Read the model definition and answer for the solid it produces. Units are mm, in the model's axes. A direction names the side the tool comes from. Coordinates: 2 decimals unless noted, no trailing zeros. Order: outer loops, then holes, each group sorted by start corner. A loop starts at its lowest first (then second) coordinate and runs counter-clockwise, first axis right, second up. Notation, with made-up numbers: (74.5, 67) -> (82.5, 67) arc R5 cw to (82.5, 72) -> close; hole circle Ø10 at (-5, 60.25). An arc over 180 degrees is marked (long way). Return JSON: item names as keys, results as strings. Group by question number.
```python
from build123d import *

# Parameters (mm, degrees)
SKETCH1_R                                       = 28.5
BOSS_EXTRUDE1_DEPTH                             = 33
SHELL1_T                                        = -3
SKETCH2_W                                       = 68.33882079
SKETCH2_H                                       = 10.979214438
CUT_EXTRUDE1_DEPTH                              = 53.091266063
SKETCH3_W                                       = 40.58739611
SKETCH3_H                                       = 33
BOSS_EXTRUDE2_DEPTH                             = 30
CUT_EXTRUDE4_REACH                              = 68.35
SKETCH6_R                                       = 1.3
CIRPATTERN1_COUNT                               = 6
FILLET1_R                                       = 10
SHELL2_START                                    = 10
SHELL2_DEPTH                                    = 13
SKETCH9_W                                       = 16.58739611
SKETCH9_H                                       = 5.010392781
CUT_EXTRUDE6_DEPTH                              = 12
CSK_FOR_M3_FLAT_HEAD_MACHINE_SCREW1_D           = 3.2
CSK_FOR_M3_FLAT_HEAD_MACHINE_SCREW1_DEPTH       = 10
CSK_FOR_M3_FLAT_HEAD_MACHINE_SCREW1_CSINK_D     = 6.3
CSK_FOR_M3_FLAT_HEAD_MACHINE_SCREW1_CSINK_ANGLE = 90
CSK_FOR_M3_FLAT_HEAD_MACHINE_SCREW1_TIP         = 0.96137699
FILLET2_R                                       = 5
FILLET3_R                                       = 5


# Read off the part's stored shape, not the designer's step: Shell2
with BuildPart() as part:
    # Sketch1 → Boss-Extrude1 (new body)
    with BuildSketch(Plane.XY):
        Circle(SKETCH1_R)
    extrude(amount=BOSS_EXTRUDE1_DEPTH)

    # Shell1
    shell1_openings = [part.faces().sort_by_distance(p)[0] for p in [
        (0, 0, 33),
    ]]
    offset(amount=SHELL1_T, openings=shell1_openings, kind=Kind.INTERSECTION)

    # Sketch2 → Cut-Extrude1 (cut, through all)
    with BuildSketch(Plane.XY.offset(33)):
        with Locations((0, 25.5)):
            Rectangle(SKETCH2_W, SKETCH2_H)
    extrude(amount=-CUT_EXTRUDE1_DEPTH, mode=Mode.SUBTRACT)

    # Sketch3 → Boss-Extrude2 (add)
    with BuildSketch(Plane(origin=(0, 20.010392781, 0), x_dir=(1, 0, 0), z_dir=(0, 1, 0))):
        with Locations((0, -16.5)):
            Rectangle(SKETCH3_W, SKETCH3_H)
    extrude(amount=BOSS_EXTRUDE2_DEPTH)

    # Sketch6 → Cut-Extrude4 (cut, up to next)
    with BuildSketch(Plane(origin=(0, 0, 0), x_dir=(-1, 0, 0), z_dir=(0, 0, -1)), mode=Mode.PRIVATE) as cut_extrude4_sk1:
        with Locations((0, -22.5)):
            Circle(SKETCH6_R)
    cut_extrude4_tool1 = extrude(cut_extrude4_sk1.sketch, amount=-CUT_EXTRUDE4_REACH, mode=Mode.PRIVATE) & part.part
    cut_extrude4 = cut_extrude4_tool1.solids().sort_by_distance((0, -22.5, 0))[0]
    add(cut_extrude4, mode=Mode.SUBTRACT)

    # CirPattern1: Cut-Extrude4 ×6 about axis, 1 skipped
    cirpattern1_axis = Axis((0, 0, 0), (0, 0, 1))
    add([cut_extrude4.rotate(cirpattern1_axis, i * 360 / CIRPATTERN1_COUNT) for i in range(1, CIRPATTERN1_COUNT) if i not in (3,)], mode=Mode.SUBTRACT)

    # Fillet1
    fillet1_edges = [part.edges().sort_by_distance(p)[0] for p in [
        (-20.293698055, 20.010392781, 16.5),
        (20.293698055, 20.010392781, 16.5),
        (-20.293698055, 50.010392781, 16.5),
        (20.293698055, 50.010392781, 16.5),
    ]]
    fillet(fillet1_edges, radius=FILLET1_R)

    # Shell2 outline → Shell2 (cut)
    with BuildSketch(Plane.XY.offset(SHELL2_START)):
        with BuildLine():
            Line((-10.293698055, 40.010392781), (-10.293698055, 23.760089607))
            ThreePointArc((-10.293698055, 23.760089607), (-10.382557976, 21.876874075), (-10.648348129, 20.010392781))
            Line((-10.648348129, 20.010392781), (10.648348129, 20.010392781))
            ThreePointArc((10.648348129, 20.010392781), (10.382557976, 21.876874075), (10.293698055, 23.760089607))
            Line((10.293698055, 23.760089607), (10.293698055, 40.010392781))
            Line((10.293698055, 40.010392781), (-10.293698055, 40.010392781))
        make_face()
    extrude(amount=SHELL2_DEPTH, mode=Mode.SUBTRACT)

    # Sketch9 → Cut-Extrude6 (cut)
    with BuildSketch(Plane(origin=(0, 0, 0), x_dir=(-1, 0, 0), z_dir=(0, 0, -1))):
        with Locations((0, 32.505196391)):
            Rectangle(SKETCH9_W, SKETCH9_H)
    extrude(amount=-CUT_EXTRUDE6_DEPTH, mode=Mode.SUBTRACT)

    # CSK for M3 Flat Head Machine Screw1
    with Locations(Plane(origin=(0, 0, 0), x_dir=(-1, 0, 0), z_dir=(0, 0, -1))):
        with Locations((-14, 43.010392781), (-14, 29.010392781), (14, 43.010392781), (14, 36.010392781), (14, 29.010392781), (-14, 36.010392781)):
            CounterSinkHole(CSK_FOR_M3_FLAT_HEAD_MACHINE_SCREW1_D / 2, CSK_FOR_M3_FLAT_HEAD_MACHINE_SCREW1_CSINK_D / 2, depth=CSK_FOR_M3_FLAT_HEAD_MACHINE_SCREW1_DEPTH, counter_sink_angle=CSK_FOR_M3_FLAT_HEAD_MACHINE_SCREW1_CSINK_ANGLE)
            with Locations((0, 0, -(CSK_FOR_M3_FLAT_HEAD_MACHINE_SCREW1_DEPTH + CSK_FOR_M3_FLAT_HEAD_MACHINE_SCREW1_TIP / 2))):  # 118° drill point
                Cone(0, CSK_FOR_M3_FLAT_HEAD_MACHINE_SCREW1_D / 2, CSK_FOR_M3_FLAT_HEAD_MACHINE_SCREW1_TIP, mode=Mode.SUBTRACT)

    # Fillet2
    fillet2_edges = [part.edges().sort_by_distance(p)[0] for p in [
        (0, 20.010392781, 23),
        (0, 20.010392781, 10),
        (10.648348129, 20.010392781, 16.5),
        (-10.648348129, 20.010392781, 16.5),
    ]]
    fillet(fillet2_edges, radius=FILLET2_R)

    # Fillet3
    # the kernel refuses this fillet: 5 mm, written as the material it takes off along each edge
    with BuildSketch(Plane(origin=(-8.293698055, 30, 10), x_dir=(0, -1, 0), z_dir=(1, 0, 0))) as fillet3_piece_1:
        with BuildLine():
            CenterArc((FILLET3_R, FILLET3_R), FILLET3_R, 180, 90)
            Line((0, FILLET3_R), (0, 0))
            Line((0, 0), (FILLET3_R, 0))
        make_face()
    extrude(amount=16.58739611, mode=Mode.SUBTRACT)


solid = part.part
```
1. Given pin 1 (18 mm diameter, centred on y = 33.5, z = 23.5, fed in from -X); pin 2 (11 mm diameter, centred on y = 28, z = 5, fed in from +X); pin 3 (2 mm diameter, centred on y = -16, z = 16.5, fed in from +X), each flat-ended and moving along its own axis, determine where each tip first touches the part or whether it passes through.
2. Straight lines are drawn through the part: L1, parallel to Y at x = 0, z = 21; L2, parallel to Y at x = 0, z = 1.65; L3, parallel to X at y = -20, z = 16.5. For each, find the intervals that lie inside material, in ascending order.
3. Find section B-B on x = -4. Determine the outline of the cut face in (y, z), and give its area (3 significant figures).
4. Find section D-D on y = 8. Determine the outline of the cut face in (x, z).
5. Find section C-C on x = -23.5. Determine the outline of the cut face in (y, z).
6. For a pull along X with two mould halves and no side action, classify faces 4 (the face through (17.287, 47.159, 16.269)), 5 (the face through (0, 29, 8)), 6 (the face through (-20.826, 20.54, 16.269)) as released by +X, released by -X, zero draft, split by the parting line, or undercut.
7. Find section A-A on y = -22.5. Determine the outline of the cut face in (x, z).
8. Which of the six approach directions +Z, -Z, +X, -X, +Y, -Y give full straight-line access (tool end or side, diameter ignored) to faces 1 (the face through (13.65, 34.45, 5.83)), 2 (the face through (18.246, 11.64, 1.479)), 3 (the face through (0, 33, 23))?
Result:
{
 "1": {"pin 1": "x = -20.29", "pin 2": "x = 20.37", "pin 3": "x = 24.23"},
 "2": {"L1": "-28.5 to -25.5, 40.01 to 50.01", "L2": "-28.5 to -23.8, -21.2 to 30, 35.01 to 50.01", "L3": "-20.3 to -15.82, 15.82 to 20.3"},
 "3": {"outline": "(-28.22, 0) -> (30, 0) -> (30, 5) arc R5 ccw to (25.01, 10) arc R5 ccw to (20.01, 5) -> (20.01, 3) -> (-25.18, 3) -> (-25.18, 33) -> (-28.22, 33) -> close; (20.01, 28) arc R5 ccw to (25.01, 23) -> (40.01, 23) -> (40.01, 10) -> (35.01, 10) -> (35.01, 0) -> (50.01, 0) -> (50.01, 33) -> (20.01, 33) -> close", "area": "899 mm^2"},
 "4": {"outline": "(-27.35, 0) -> (27.35, 0) -> (27.35, 33) -> (24.21, 33) -> (24.21, 3) -> (-24.21, 3) -> (-24.21, 33) -> (-27.35, 33) -> close"},
 "5": {"outline": "(-16.12, 0) -> (16.12, 0) -> (16.12, 33) -> (9.9, 33) -> (9.9, 3) -> (-9.9, 3) -> (-9.9, 33) -> (-16.12, 33) -> close"},
 "6": {"face 4": "released by +X", "face 5": "undercut", "face 6": "released by -X"},
 "7": {"outline": "(-17.49, 0) -> (-1.3, 0) -> (-1.3, 3) -> (-12, 3) -> (-12, 33) -> (-17.49, 33) -> close; (1.3, 0) -> (17.49, 0) -> (17.49, 33) -> (12, 33) -> (12, 3) -> (1.3, 3) -> close"},
 "8": {"face 1": "-Z", "face 2": "+Z, -Z", "face 3": "none"}
}
